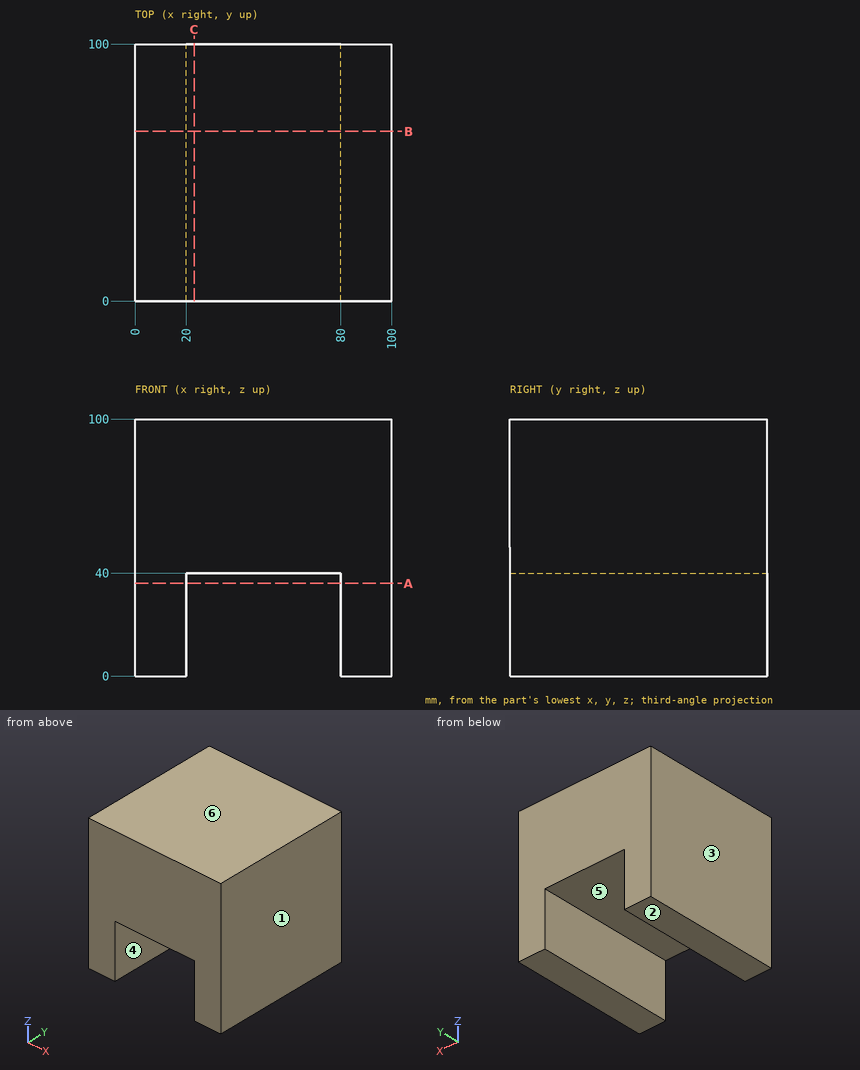
Here's the drawing with two shaded views (mm, measured from the low corner). I have some questions. A direction names the side the tool comes from. Give positions to 0.01 mm unless a question says otherwise; leave off trailing zeros. Loops run counter-clockwise (first coordinate to the right, second up) from the corner with the lowest first, then second, coordinate; pieces in that order, holes last. Notation, with made-up numbers: (19.5, 37.25) -> (60.5, 37.25) arc R37 cw to (60.5, 74.25) -> close; hole circle Ø2 at (-7.75, 1). An arc over 180 degrees is marked (long way). Answer as a JSON object with one key per item and string values. Group by question number.
Item 1: Thinking about a two-plate mould opening in X: for the marked faces 1, 2, 3 and 4, which applies, pulls with the +X half, pulls with the -X half, needs draft (parallel to the pull), parting line crosses it, or undercut?
Item 2: On a 3-axis mill with a long thin cutter (end or side, diameter ignored), from which of +Z, -Z, +X, -X, +Y, -Y can I reach the whole of each face in a straight line? I mean the marked faces 5 and 6. Say none if no direction works.
Item 3: Imagine slicing it at C-C on x = 23. Write out the boundary of the cut face in (y, z), then the cut area to 3 significant figures.
Item 4: Will this pin go through, and if not, where does the flat tip stop? pin 1 (4 mm diameter, centred on x = 52, y = 52.5, fed in from -Z).
Item 5: Imagine slicing it at B-B on y = 66. Write out the boundary of the cut face in (x, z).
Item 6: I need wall thicknesses on L1, parallel to X at y = 64, z = 13.5; L2, parallel to Z at x = 70, y = 12. Which ranges of each line are inside material? Lowest first, please.
Item 7: Imagine slicing it at A-A on z = 36. Write out the boundary of the cut face in (x, y).
Answer list:
{
 "1": {"face 1": "pulls with the +X half", "face 2": "needs draft", "face 3": "pulls with the -X half", "face 4": "undercut"},
 "2": {"face 5": "-Z, +Y, -Y", "face 6": "+Z, +X, -X, +Y, -Y"},
 "3": {"outline": "(0, 40) -> (100, 40) -> (100, 100) -> (0, 100) -> close", "area": "6,000 mm2"},
 "4": {"pin 1": "stops at z = 40"},
 "5": {"outline": "(0, 0) -> (20, 0) -> (20, 40) -> (80, 40) -> (80, 0) -> (100, 0) -> (100, 100) -> (0, 100) -> close"},
 "6": {"L1": "x = 0 to 20, 80 to 100", "L2": "z = 40 to 100"},
 "7": {"outline": "(0, 0) -> (20, 0) -> (20, 100) -> (0, 100) -> close; (80, 0) -> (100, 0) -> (100, 100) -> (80, 100) -> close"}
}
